from build123d import *

# Parameters (mm, degrees)
PAD_DEPTH    = 120
SKETCH001_R  = 10
PAD001_DEPTH = 40
FILLET_R     = 1
SKETCH002_W  = 35
SKETCH002_H  = 30
PAD002_DEPTH = 22
FILLET001_R  = 10
FILLET002_R  = 4


with BuildPart() as part:
    # Sketch → Pad (new body)
    with BuildSketch(Plane.XY):
        with BuildLine():
            Line((-35, 43.30686), (35, 43.30686))
            ThreePointArc((40, 38.30686), (38.535534, 41.842393), (35, 43.30686))
            Line((40, 38.30686), (40, -31.69314))
            ThreePointArc((35, -36.69314), (38.535534, -35.228674), (40, -31.69314))
            Line((35, -36.69314), (-35, -36.69314))
            ThreePointArc((-40, -31.69314), (-38.535534, -35.228674), (-35, -36.69314))
            Line((-40, -31.69314), (-40, 38.30686))
            ThreePointArc((-35, 43.30686), (-38.535534, 41.842393), (-40, 38.30686))
        make_face()
    extrude(amount=PAD_DEPTH)

    # Sketch001 (on Face10 of Pad) → Pad001 (join)
    with BuildSketch(Plane.XY.offset(120)):
        Circle(SKETCH001_R)
    extrude(amount=PAD001_DEPTH)

    # Fillet
    fillet_edges = [part.edges().sort_by_distance(p)[0] for p in [
        (-10, 0, 160),
    ]]
    fillet(fillet_edges, radius=FILLET_R)

    # Sketch002 (on Face8 of Fillet) → Pad002 (join)
    with BuildSketch(Plane(origin=(-40, 0, 0), x_dir=(0, -1, 0), z_dir=(-1, 0, 0))):
        with Locations((0, 15)):
            Rectangle(SKETCH002_W, SKETCH002_H)
    extrude(amount=PAD002_DEPTH)

    # Fillet001
    fillet001_edges = [part.edges().sort_by_distance(p)[0] for p in [
        (-62, 17.5, 15),
        (-62, -17.5, 15),
    ]]
    fillet(fillet001_edges, radius=FILLET001_R)

    # Fillet002
    fillet002_edges = [part.edges().sort_by_distance(p)[0] for p in [
        (-62, 0, 0),
    ]]
    fillet(fillet002_edges, radius=FILLET002_R)


solid = part.part
The model under review builds one solid part; all positions refer to its coordinate system, in mm. A direction names the side the tool comes from. Give positions to 0.01 mm unless a question says otherwise; leave off trailing zeros. Order: outer loops, then holes, each group sorted by start corner. A loop starts at its lowest first (then second) coordinate and runs counter-clockwise, first axis right, second up. Notation, with made-up numbers: M 39,75 L 44,75 A23 cw 44,90 Z; hole C 2,72.5 d6. An arc over 180 degrees is marked long. Use one line per item in the form item = value. Start each with the question number.
Item 1: We need section A-A on y = 0. Give the boundary of the cut face in (x, z), plus the area to 3 significant figures.
Item 2: We need section B-B on z = 87.5. Give the boundary of the cut face in (x, y), plus the area to 3 significant figures.
Item 3: To check wall thickness, follow line 1 along X through (y, z) = (32, 15.5); line 2 along Z through (x, y) = (-38, -13); line 3 along Y through (x, z) = (36, 118). State the ranges of each line that lie inside material, in increasing order. Write a range as from..to.
Item 4: We need section C-C on x = 0. Give the boundary of the cut face in (y, z).
Item 5: Insertion check: pin 1 Ø6 at (x, z) = (-47.5, 13) entering from -Y; pin 2 Ø11 at (x, y) = (-55.5, 7.5) entering from +Z; pin 3 Ø4 at (x, z) = (9, 144) entering from -Y. Each pin has a flat end and moves straight along its axis. Give the tip position at first contact, or say it passes through.
Item 6: We need section D-D on z = 26. Give the boundary of the cut face in (x, y), plus the area to 3 significant figures.
Item 7: For faces 1 (the cylindrical face through (-2.17, -9.76, 139.23)), 2 (the flat face through (-46, 17.5, 17)), 3 (the flat face through (-46, -17.5, 17)), 4 (the cylindrical face through (-45.916, -16.297, 1.141)), list the 3-axis set-ups (+Z, -Z, +X, -X, +Y, -Y) from which the entire face can be reached by the end or side of a thin tool; tool diameter is ignored.
Completed:
q1.outline = M -62,4 A4 ccw -58,0 L 40,0 L 40,120 L 10,120 L 10,159 A1 ccw 9,160 L -9,160 A1 ccw -10,159 L -10,120 L -40,120 L -40,30 L -62,30 Z
q1.area = 11,100 mm²
q2.outline = M -40,-31.69 A5 ccw -35,-36.69 L 35,-36.69 A5 ccw 40,-31.69 L 40,38.31 A5 ccw 35,43.31 L -35,43.31 A5 ccw -40,38.31 Z
q2.area = 6,380 mm²
q3.line_1 = -40..40
q3.line_2 = 0..120
q3.line_3 = -36.59..43.21
q4.outline = M -36.69,0 L 43.31,0 L 43.31,120 L 10,120 L 10,159 A1 ccw 9,160 L -9,160 A1 ccw -10,159 L -10,120 L -36.69,120 Z
q5.pin_1 = -17.5
q5.pin_2 = 30
q5.pin_3 = -7.14
q6.outline = M -62,-7.5 A10 ccw -52,-17.5 L -40,-17.5 L -40,-31.69 A5 ccw -35,-36.69 L 35,-36.69 A5 ccw 40,-31.69 L 40,38.31 A5 ccw 35,43.31 L -35,43.31 A5 ccw -40,38.31 L -40,17.5 L -52,17.5 A10 ccw -62,7.5 Z
q6.area = 7,110 mm²
q7.face_1 = +Z
q7.face_2 = +Z, -Z, -X, +Y
q7.face_3 = +Z, -Z, -X, -Y
q7.face_4 = -Z, -X, -Y
